Verification items for this drawing (mm, ordinates from the low corner). Round coordinates to 2 decimals unless told otherwise and drop trailing zeros. Order: outer loops, then holes, each group sorted by start corner. A loop starts at its lowest first (then second) coordinate and runs counter-clockwise, first axis right, second up. Notation, with made-up numbers: (-2.75, -19.5) - (42.25, -19.5) arc R8 cw to (42.25, -4.5) - close; hole circle Ø10 at (-24, -1.5). An arc over 180 degrees is marked (long way). Use a Markdown table: item, result. Add a question column.
(1) Section check C-C on x = 35. Record the boundary of the cut face in (y, z).
(2) Thickness scan on line 1 along X through (y, z) = (4.75, 14); line 2 along X through (y, z) = (7, 14.5) (1 decimal); line 3 along X through (y, z) = (5.25, 27). Record the ranges inside material, lowest first. Write a range as [from, to].
(3) Section check D-D on x = 22. Record the boundary of the cut face in (y, z) (1 decimal).
(4) Section check A-A on z = 8. Record the boundary of the cut face in (x, y) (1 decimal), then the cut area to 3 significant figures.
(5) Mould release check, pull along X, two halves, no side actions. Record for the marked faces 1, 2, 3 and 4: released by +X, released by -X, zero draft, split by the parting line, or undercut.
(6) Gauge pin test, flat ends, axial feed: P1, Ø5.5, axis at x = 20.5, z = 20.5, coming from the +Y side; P2, Ø2.5, axis at x = 3, y = 3.5, coming from the +Z side; P3, Ø1.9, axis at x = 35.72, y = 4.76, coming from the +Z side; P4, Ø2.5, axis at y = 4, z = 38.5, coming from the +X side. Record the tip position at first contact, or that the pin passes through.
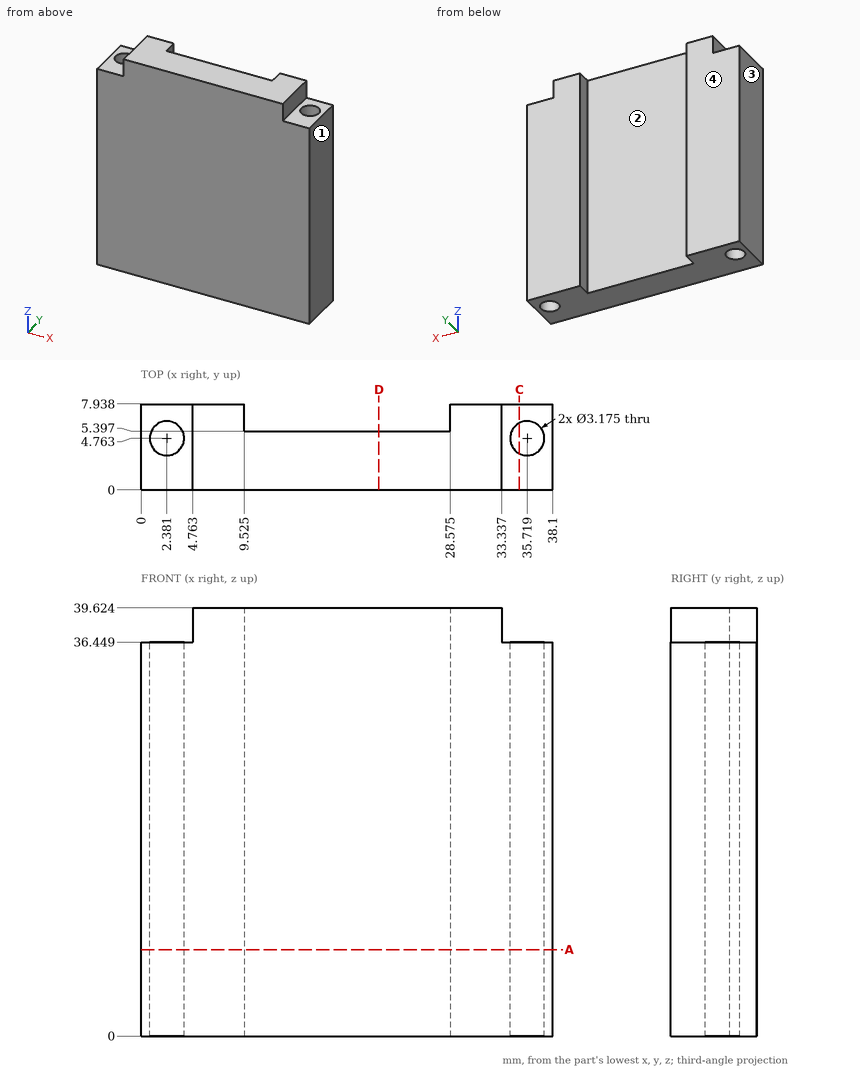
Check sheet entries:
| question | item | result |
|---|---|---|
| 1 | outline | (0, 0) - (3.35, 0) - (3.35, 36.45) - (0, 36.45) - close; (6.18, 0) - (7.94, 0) - (7.94, 36.45) - (6.18, 36.45) - close |
| 2 | line 1 | x = [0, 0.79], [3.97, 34.13], [37.31, 38.1] |
| 2 | line 2 | x = [0, 9.5], [28.6, 38.1] |
| 2 | line 3 | x = [0, 0.87], [3.89, 34.21], [37.23, 38.1] |
| 3 | outline | (0, 0) - (5.4, 0) - (5.4, 39.6) - (0, 39.6) - close |
| 4 | outline | (0, 0) - (38.1, 0) - (38.1, 7.9) - (28.6, 7.9) - (28.6, 5.4) - (9.5, 5.4) - (9.5, 7.9) - (0, 7.9) - close; hole circle Ø3.2 at (2.4, 4.8); hole circle Ø3.2 at (35.7, 4.8) |
| 4 | area | 238 mm2 |
| 5 | face 1 | released by +X |
| 5 | face 2 | undercut |
| 5 | face 3 | released by -X |
| 5 | face 4 | zero draft |
| 6 | P1 | stops at y = 5.4 |
| 6 | P2 | stops at z = 36.45 |
| 6 | P3 | passes through |
| 6 | P4 | stops at x = 33.34 |
